Here's the drawing with two shaded views (mm, measured from the low corner). I have some questions. Coordinates: 2 decimals unless noted, no trailing zeros. Write each loop counter-clockwise with the first axis right and the second up, starting at its lowest first coordinate (ties: lowest second). Pieces come first, ordered by that corner, then holes.
Item 1: If we section it at C-C (y = 4.5): Please give me the cut outline in (x, z) (1 decimal), then the cut area to 3 significant figures.
Item 2: If we section it at A-A (z = 0.9): Please give me the cut outline in (x, y) (1 decimal).
Item 3: If we section it at B-B (x = 42): Please give me the cut outline in (y, z) (1 decimal), then the cut area to 3 significant figures.
Item 4: If I drill on line 1 (Y direction, x = 31.5, z = 2.7) (1 decimal); line 2 (X direction, y = 33, z = 0.35) (1 decimal), over which ranges is the centre line in solid material (lowest first)?
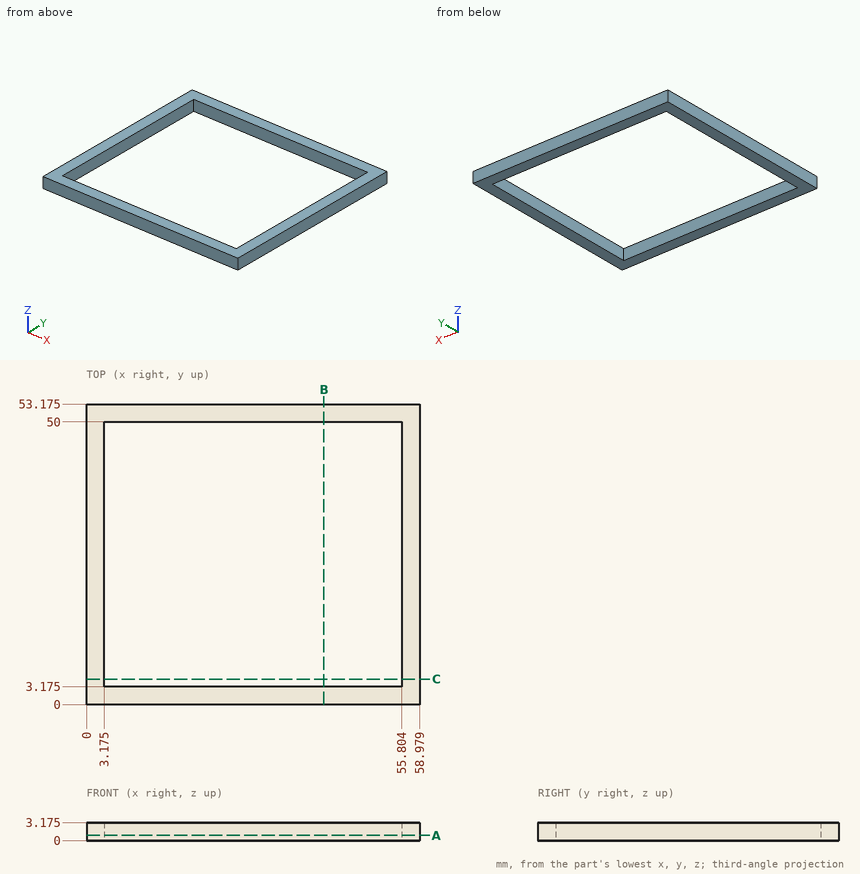
Answer list:
1. outline: (0, 0) - (3.2, 0) - (3.2, 3.2) - (0, 3.2) - close; (55.8, 0) - (59, 0) - (59, 3.2) - (55.8, 3.2) - close
1. area: 20.2 mm2
2. outline: (0, 0) - (59, 0) - (59, 53.2) - (0, 53.2) - close; hole (3.2, 3.2) - (55.8, 3.2) - (55.8, 50) - (3.2, 50) - close
3. outline: (0, 0) - (3.2, 0) - (3.2, 3.2) - (0, 3.2) - close; (50, 0) - (53.2, 0) - (53.2, 3.2) - (50, 3.2) - close
3. area: 20.2 mm2
4. line 1: y = 0 to 3.2, 50 to 53.2
4. line 2: x = 0 to 3.2, 55.8 to 59
